Can you work these out from the model? Positions are in its coordinate system, mm. Coordinates: 2 decimals unless noted, no trailing zeros. Write each loop counter-clockwise with the first axis right and the second up, starting at its lowest first coordinate (ties: lowest second). Pieces come first, ordered by that corner, then holes.
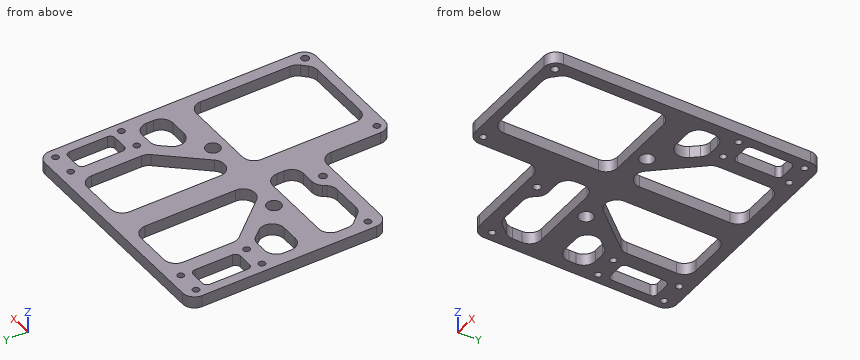
```python
from build123d import *

# Parameters (mm, degrees)
SKETCH_1_R      = 1.4
SKETCH_1_R_2    = 3
SKETCH_1_R_3    = 1.6
EXTRUDE_1_DEPTH = 5


with BuildPart() as part:
    # ｽｹｯﾁ1 → ﾎﾞｽ - 押し出し1 (new body)
    with BuildSketch(Plane.XY):
        with BuildLine():
            Line((-45, 57.5), (45, 57.5))
            ThreePointArc((45, 57.5), (48.535533906, 56.035533906), (50, 52.5))
            Line((50, 52.5), (50, -52.5))
            ThreePointArc((50, -52.5), (48.535533906, -56.035533906), (45, -57.5))
            Line((45, -57.5), (0, -57.5))
            ThreePointArc((0, -57.5), (-3.535533906, -56.035533906), (-5, -52.5))
            Line((-5, -52.5), (-5, -31.5))
            ThreePointArc((-5, -31.5), (-6.464466094, -27.964466094), (-10, -26.5))
            Line((-10, -26.5), (-45, -26.5))
            ThreePointArc((-45, -26.5), (-48.535533906, -25.035533906), (-50, -21.5))
            Line((-50, -21.5), (-50, 52.5))
            ThreePointArc((-50, 52.5), (-48.535533906, 56.035533906), (-45, 57.5))
        make_face()
        with Locations((-46, 52.5)):
            Circle(SKETCH_1_R, mode=Mode.SUBTRACT)
        with Locations((-36, 52.5)):
            Circle(SKETCH_1_R, mode=Mode.SUBTRACT)
        with Locations((-46, 24.5)):
            Circle(SKETCH_1_R, mode=Mode.SUBTRACT)
        with Locations((-36, 24.5)):
            Circle(SKETCH_1_R, mode=Mode.SUBTRACT)
        with Locations((46, 24.5)):
            Circle(SKETCH_1_R, mode=Mode.SUBTRACT)
        with Locations((36, 24.5)):
            Circle(SKETCH_1_R, mode=Mode.SUBTRACT)
        with Locations((36, 52.5)):
            Circle(SKETCH_1_R, mode=Mode.SUBTRACT)
        with Locations((46, 52.5)):
            Circle(SKETCH_1_R, mode=Mode.SUBTRACT)
        with Locations((-20, 2.5)):
            Circle(SKETCH_1_R_2, mode=Mode.SUBTRACT)
        with Locations((20, 2.5)):
            Circle(SKETCH_1_R_2, mode=Mode.SUBTRACT)
        with Locations((-1, -53.5)):
            Circle(SKETCH_1_R, mode=Mode.SUBTRACT)
        with Locations((-46, -20.5)):
            Circle(SKETCH_1_R, mode=Mode.SUBTRACT)
        with Locations((46, -53.5)):
            Circle(SKETCH_1_R_3, mode=Mode.SUBTRACT)
        with Locations((-15, -21.5)):
            Circle(SKETCH_1_R_3, mode=Mode.SUBTRACT)
        with BuildLine():
            Line((-10, 52.5), (-25, 52.5))
            ThreePointArc((-25, 52.5), (-28.535533906, 51.035533906), (-30, 47.5))
            Line((-30, 47.5), (-30, 26.369875327))
            ThreePointArc((-30, 26.369875327), (-29.683222077, 24.618467044), (-28.773027611, 23.088981752))
            Line((-28.773027611, 23.088981752), (-13.773027611, 5.838981752))
            ThreePointArc((-13.773027611, 5.838981752), (-8.248591717, 4.43665325), (-5, 9.119875327))
            Line((-5, 9.119875327), (-5, 47.5))
            ThreePointArc((-5, 47.5), (-6.464466094, 51.035533906), (-10, 52.5))
        make_face(mode=Mode.SUBTRACT)
        with BuildLine():
            Line((-40, 19.5), (-35.318994756, 19.5))
            ThreePointArc((-35.318994756, 19.5), (-33.215254758, 19.035887787), (-31.502063329, 17.729711207))
            Line((-31.502063329, 17.729711207), (-28.963601791, 14.729711207))
            ThreePointArc((-28.963601791, 14.729711207), (-28.24464543, 9.396260001), (-32.780533218, 6.5))
            Line((-32.780533218, 6.5), (-40, 6.5))
            ThreePointArc((-40, 6.5), (-43.535533906, 7.964466094), (-45, 11.5))
            Line((-45, 11.5), (-45, 14.5))
            ThreePointArc((-45, 14.5), (-43.535533906, 18.035533906), (-40, 19.5))
        make_face(mode=Mode.SUBTRACT)
        with BuildLine():
            Line((-40, -3.5), (-10, -3.5))
            ThreePointArc((-10, -3.5), (-6.464466094, -4.964466094), (-5, -8.5))
            Line((-5, -8.5), (-5, -11.5))
            ThreePointArc((-5, -11.5), (-6.464466094, -15.035533906), (-10, -16.5))
            Line((-10, -16.5), (-15.596875763, -16.5))
            ThreePointArc((-15.596875763, -16.5), (-17.762819415, -16.993483818), (-19.50121981, -18.376524762))
            Line((-19.50121981, -18.376524762), (-20.49878019, -19.623475238))
            ThreePointArc((-20.49878019, -19.623475238), (-22.237180585, -21.006516182), (-24.403124237, -21.5))
            Line((-24.403124237, -21.5), (-36.497595845, -21.5))
            ThreePointArc((-36.497595845, -21.5), (-38.537567248, -21.064922417), (-40.222520321, -19.835406669))
            Line((-40.222520321, -19.835406669), (-43.724924476, -15.923982291))
            ThreePointArc((-43.724924476, -15.923982291), (-44.670365209, -14.373985605), (-45, -12.588575621))
            Line((-45, -12.588575621), (-45, -8.5))
            ThreePointArc((-45, -8.5), (-43.535533906, -4.964466094), (-40, -3.5))
        make_face(mode=Mode.SUBTRACT)
        with BuildLine():
            Line((40, 6.5), (32.780533218, 6.5))
            ThreePointArc((32.780533218, 6.5), (28.24464543, 9.396260001), (28.963601791, 14.729711207))
            Line((28.963601791, 14.729711207), (31.502063329, 17.729711207))
            ThreePointArc((31.502063329, 17.729711207), (33.215254758, 19.035887787), (35.318994756, 19.5))
            Line((35.318994756, 19.5), (40, 19.5))
            ThreePointArc((40, 19.5), (43.535533906, 18.035533906), (45, 14.5))
            Line((45, 14.5), (45, 11.5))
            ThreePointArc((45, 11.5), (43.535533906, 7.964466094), (40, 6.5))
        make_face(mode=Mode.SUBTRACT)
        with BuildLine():
            Line((-44, 48.5), (-38, 48.5))
            ThreePointArc((-38, 48.5), (-36.585786438, 47.914213562), (-36, 46.5))
            Line((-36, 46.5), (-36, 30.5))
            ThreePointArc((-36, 30.5), (-36.585786438, 29.085786438), (-38, 28.5))
            Line((-38, 28.5), (-44, 28.5))
            ThreePointArc((-44, 28.5), (-45.414213562, 29.085786438), (-46, 30.5))
            Line((-46, 30.5), (-46, 46.5))
            ThreePointArc((-46, 46.5), (-45.414213562, 47.914213562), (-44, 48.5))
        make_face(mode=Mode.SUBTRACT)
        with BuildLine():
            Line((30, 47.5), (30, 26.369875327))
            ThreePointArc((30, 26.369875327), (29.683222077, 24.618467044), (28.773027611, 23.088981752))
            Line((28.773027611, 23.088981752), (13.773027611, 5.838981752))
            ThreePointArc((13.773027611, 5.838981752), (8.248591717, 4.43665325), (5, 9.119875327))
            Line((5, 9.119875327), (5, 47.5))
            ThreePointArc((5, 47.5), (6.464466094, 51.035533906), (10, 52.5))
            Line((10, 52.5), (25, 52.5))
            ThreePointArc((25, 52.5), (28.535533906, 51.035533906), (30, 47.5))
        make_face(mode=Mode.SUBTRACT)
        with BuildLine():
            Line((44, 28.5), (38, 28.5))
            ThreePointArc((38, 28.5), (36.585786438, 29.085786438), (36, 30.5))
            Line((36, 30.5), (36, 46.5))
            ThreePointArc((36, 46.5), (36.585786438, 47.914213562), (38, 48.5))
            Line((38, 48.5), (44, 48.5))
            ThreePointArc((44, 48.5), (45.414213562, 47.914213562), (46, 46.5))
            Line((46, 46.5), (46, 30.5))
            ThreePointArc((46, 30.5), (45.414213562, 29.085786438), (44, 28.5))
        make_face(mode=Mode.SUBTRACT)
        with BuildLine():
            Line((10, -3.5), (40, -3.5))
            ThreePointArc((40, -3.5), (43.535533906, -4.964466094), (45, -8.5))
            Line((45, -8.5), (45, -46.428932188))
            ThreePointArc((45, -46.428932188), (44.619397663, -48.34234935), (43.535533906, -49.964466094))
            Line((43.535533906, -49.964466094), (41.464466094, -52.035533906))
            ThreePointArc((41.464466094, -52.035533906), (39.84234935, -53.119397663), (37.928932188, -53.5))
            Line((37.928932188, -53.5), (10, -53.5))
            ThreePointArc((10, -53.5), (6.464466094, -52.035533906), (5, -48.5))
            Line((5, -48.5), (5, -8.5))
            ThreePointArc((5, -8.5), (6.464466094, -4.964466094), (10, -3.5))
        make_face(mode=Mode.SUBTRACT)
    extrude(amount=EXTRUDE_1_DEPTH)


solid = part.part
```
1. I'm going to push flat-ended pins straight in: P1, Ø1, axis at y = -40, z = 2, coming from the -X side; P2, Ø2.5, axis at x = -15.5, z = 1.5, coming from the -Y side. Where does each tip first touch, or does it pass through?
2. If we section it at B-B, the plane y = -37: List the corners of the cut face in (x, z) for me.
3. If we section it at D-D, the plane y = -14.5: List the corners of the cut face in (x, z) for me, plus the area to 3 significant figures.
4. If we section it at A-A, the plane x = 20: List the corners of the cut face in (y, z) for me.
5. If I drill on L1, parallel to X at y = 44.5, z = 2.25; L2, parallel to X at y = -10, z = 1.85; L3, parallel to Y at x = -10, z = 0.6, over which ranges is the centre line in solid material (lowest first)?
6. If we section it at C-C, the plane y = 24.5: List the corners of the cut face in (x, z) for me, plus the area to 3 significant figures.
Answers:
1. P1: stops at x = -5
1. P2: stops at y = -26.5
2. outline: (-5, 0) - (5, 0) - (5, 5) - (-5, 5) - close; (45, 0) - (50, 0) - (50, 5) - (45, 5) - close
3. outline: (-50, 0) - (-44.62, 0) - (-44.62, 5) - (-50, 5) - close; (-6, 0) - (5, 0) - (5, 5) - (-6, 5) - close; (45, 0) - (50, 0) - (50, 5) - (45, 5) - close
3. area: 107 mm2
4. outline: (-57.5, 0) - (-53.5, 0) - (-53.5, 5) - (-57.5, 5) - close; (-3.5, 0) - (-0.5, 0) - (-0.5, 5) - (-3.5, 5) - close; (5.5, 0) - (13, 0) - (13, 5) - (5.5, 5) - close; (52.5, 0) - (57.5, 0) - (57.5, 5) - (52.5, 5) - close
5. L1: x = -50 to -46, -36 to -30, -5 to 5, 30 to 36, 46 to 50
5. L2: x = -50 to -45, -5 to 5, 45 to 50
5. L3: y = -26.5 to -16.5, -3.5 to 4.12, 52.5 to 57.5
6. outline: (-50, 0) - (-47.4, 0) - (-47.4, 5) - (-50, 5) - close; (-44.6, 0) - (-37.4, 0) - (-37.4, 5) - (-44.6, 5) - close; (-34.6, 0) - (-29.64, 0) - (-29.64, 5) - (-34.6, 5) - close; (-5, 0) - (5, 0) - (5, 5) - (-5, 5) - close; (29.64, 0) - (34.6, 0) - (34.6, 5) - (29.64, 5) - close; (37.4, 0) - (44.6, 0) - (44.6, 5) - (37.4, 5) - close; (47.4, 0) - (50, 0) - (50, 5) - (47.4, 5) - close
6. area: 198 mm2
